Autodesk Inventor part; units mm, degrees
ref_plane "YZ Plane" through (0, 0, 0) normal (1, 0, 0) x (0, 1, 0)
ref_plane "XZ Plane" through (0, 0, 0) normal (0, 1, 0) x (-1, 0, 0)
ref_plane "XY Plane" through (0, 0, 0) normal (0, 0, 1) x (1, 0, 0)
sketch "Sketch1" plane through (0, 0, 0) normal (0, 1, 0) x (-1, 0, 0)
  circle A0 centre (-3.9982, 7.6265) radius 3
  circle A1 centre (-3.9982, 7.6265) radius 5
  line L0 (-3.9982, 12.6265) -> (-8.9982, 12.6265)
  line L1 (-8.9982, 12.6265) -> (-8.9982, 2.6265)
  line L2 (-8.9982, 2.6265) -> (-3.9982, 2.6265)
  line L3 (-3.9982, 2.6265) -> (-3.9982, 12.6265)
  point P0 (0, 0)
  dimension "d0" = 6
  dimension "d1" = 2
  dimension "d8" = 0
extrude "Extrusion1" add sketch "Sketch1" along normal blind 6 contours A0 L3 A1 | A0 L3 A1
extrude "Extrusion2" add sketch "Sketch1" along normal blind 6 contours L3 A0 | A0 L3 A1 | A1 L1 L0 | L2 L1 A1 picked at (-5.8933, 7.7284) picked at (-4.3691, 3.335)
extrude "Extrusion3" cut sketch "Sketch1" along normal blind 6 contours A0 L3 | L3 A0
sketch "Sketch2" plane through (8.9982, 0, 12.6265) normal (1, 0, 0) x (0, 0, -1)
  line L0 (0, 0) -> (10, 0)
  line L1 (2, 6) -> (8, 6)
  line L2 (8, 6) -> (8, 0)
  line L3 (8, 0) -> (2, 0)
  line L4 (2, 0) -> (2, 6)
  line L5 (0, 0) -> (0, 6)
  line L6 (10, 0) -> (10, 6)
  line L7 (0, 6) -> (10, 6)
  point P0 (12.6265, 0)
  dimension "d9" = 2
  dimension "d10" = 2
extrude "Extrusion4" add sketch "Sketch2" along normal blind 45 contours L4 L1 L2 L0
chamfer "Chamfer1" distance 2 angle 45 2 edges at (8.9982, 3, 12.6265) (8.9982, 3, 2.6265)
properties part number "roka1"
Source: CAD feature listing. Evaluate the final solid. Frame: model axes, mm. A direction names the side the tool comes from. Round coordinates to 2 decimals unless told otherwise and drop trailing zeros. Order: outer loops, then holes, each group sorted by start corner. A loop starts at its lowest first (then second) coordinate and runs counter-clockwise, first axis right, second up. Notation, with made-up numbers: (-29, -24.75) - (29, -24.75) arc R13 ccw to (29, -4.75) - close; hole circle Ø6 at (-31, 58.5). An arc over 180 degrees is marked (long way). Use a Markdown table: item, result. Add a question column.
1. Section query B-B (x = 5.5). Return the cut outline in (y, z).
2. Set-up query: faces 1 (the flat face through (31, 3, 10.626)), 2 (the flat face through (31, 3, 4.626)), 3 (the flat face through (53.998, 3, 8)). Return all of +Z, -Z, +X, -X, +Y, -Y with unobstructed straight access to the full face (end or side cutting, diameter ignored); none if empty.
3. Section query D-D (x = 33.5). Return the cut outline in (y, z).
4. Line query: probe 1 along Z at (x, y) = (34.5, 3.95); probe 2 along X at (y, z) = (1, 9.5); probe 3 along X at (y, z) = (4.15, 10). Output: solid intervals per line, ascending.
5. First-contact query: pin 1 (2 mm diameter, centred on x = 33.5, y = 1.5, fed in from +Z); pin 2 (5.5 mm diameter, centred on x = 4, z = 7.63, fed in from +Y). Flat tips, straight axial feed; report the tip coordinate or a pass-through.
6. Mould query, pull axis X, two halves, no side actions, for faces 4 (the flat face through (6, 3, 2.626)), 5 (the flat face through (8.012, 3.042, 11.613)), 6 (the cylindrical face through (1.47, 2.96, 9.24)). Classes: +X half, -X half, draft (parallel to the pull), parting line (faces both ways), or undercut.
7. Section query C-C (z = 7.25). Return the cut outline in (x, y).
Derived:
| question | item | result |
|---|---|---|
| 1 | outline | (0, 2.63) - (6, 2.63) - (6, 5.03) - (0, 5.03) - close; (0, 10.22) - (6, 10.22) - (6, 12.63) - (0, 12.63) - close |
| 2 | face 1 | +Z, +X, +Y, -Y |
| 2 | face 2 | -Z, +X, +Y, -Y |
| 2 | face 3 | +Z, -Z, +X, +Y, -Y |
| 3 | outline | (0, 4.63) - (6, 4.63) - (6, 10.63) - (0, 10.63) - close |
| 4 | probe 1 | 4.63 to 10.63 |
| 4 | probe 2 | -0.64 to 1.66, 6.34 to 54 |
| 4 | probe 3 | -0.4 to 2.16, 5.83 to 54 |
| 5 | pin 1 | z = 10.63 |
| 5 | pin 2 | through |
| 6 | face 4 | draft |
| 6 | face 5 | +X half |
| 6 | face 6 | undercut |
| 7 | outline | (-0.99, 0) - (1.02, 0) - (1.02, 6) - (-0.99, 6) - close; (6.97, 0) - (54, 0) - (54, 6) - (6.97, 6) - close |
